Input: part model. Units: mm. Frame: model coordinates. A direction names the side the tool comes from. Give positions to 0.01 mm unless a question says otherwise; leave off trailing zeros. Write each loop counter-clockwise with the first axis right and the second up, starting at its lowest first coordinate (ties: lowest second). Pieces come first, ordered by that corner, then holes. Notation, with made-up numbers: (59.25, 58) - (116.25, 58) arc R27 ccw to (116.25, 97) - close; hole circle Ø9 at (12, 38.5). An arc over 180 degrees is marked (long way). Use a Markdown table: item, result. Add a question column.
1. Material intervals for probe 1 along X at (y, z) = (0.5, 0.55); probe 2 along Y at (x, z) = (0.3, -0.3); probe 3 along X at (y, z) = (5.25, 0.1), sorted ascending.
2. Set-up query: faces 4 (the flat face through (-1.3, 0, 0)), 5 (the flat face through (-0.49, 0.79, -0.87)). Return all of +Z, -Z, +X, -X, +Y, -Y with unobstructed straight access to the full face (end or side cutting, diameter ignored); none if empty.
3. Section query A-A, the plane z = 0. Return loops of the section in (x, y), plus the area to 3 significant figures.
4. Pin query (flat end, axial travel): pin 1 (3 mm diameter, centred on x = 0.5, z = -1.5, fed in from +Y); pin 2 (1.3 mm diameter, centred on y = 1, z = 0, fed in from +X). Return the tip coordinate at first contact, or that it passes through.
5. Mould query, pull axis X, two halves, no side actions, for faces 1 (the flat face through (0, 1.6, 0)), 2 (the cylindrical face through (0.06, 7.61, -1.4)), 3 (the flat face through (0, 14, 0)). Classes: released by +X, released by -X, zero draft, split by the parting line, or undercut.
6. Section query B-B, the plane y = 8. Return loops of the section in (x, z).
```python
from build123d import *

# Parameters (mm, degrees)
SKETCH_1_R      = 3
EXTRUDE_1_DEPTH = 1.6
CHAMFER_1_SIZE  = 1.6
SKETCH_2_R      = 1.4
EXTRUDE_2_DEPTH = 12.4
CHAMFER_2_SIZE  = 0.2


with BuildPart() as part:
    # 草图1 → 凸台-拉伸1 (new body)
    with BuildSketch(Plane(origin=(0, 0, 0), x_dir=(1, 0, 0), z_dir=(0, 1, 0))):
        with Locations(Location((0, 0, 0), (0, 0, 270))):
            Circle(SKETCH_1_R)
        Polygon((0, -1.154700538), (1, -0.577350269), (1, 0.577350269), (0, 1.154700538), (-1, 0.577350269), (-1, -0.577350269), align=None, mode=Mode.SUBTRACT)
    extrude(amount=EXTRUDE_1_DEPTH)

    # 倒角1
    # the kernel refuses this chamfer: 1.6 mm, written as the material it takes off along each edge
    with BuildSketch(Plane(origin=(0, 1.6, 0), x_dir=(0, 0, 1), z_dir=(-1, 0, 0))) as chamfer_1_piece_1:
        Polygon((3, -CHAMFER_1_SIZE), (3 - CHAMFER_1_SIZE, 0), (3, 0), align=None)
    revolve(axis=Axis((0, 1.6, 0), (0, 1, 0)), mode=Mode.SUBTRACT)

    # 草图2 → 凸台-拉伸2 (add)
    with BuildSketch(Plane(origin=(0, 1.6, 0), x_dir=(1, 0, 0), z_dir=(0, 1, 0))):
        with Locations(Location((0, 0, 0), (0, 0, 270))):
            Circle(SKETCH_2_R)
    extrude(amount=EXTRUDE_2_DEPTH)

    # 倒角2
    chamfer_2_edges = [part.edges().sort_by_distance(p)[0] for p in [
        (0, 14, -1.4),
    ]]
    chamfer(chamfer_2_edges, length=CHAMFER_2_SIZE)


solid = part.part
```
Result sheet:
| question | item | result |
|---|---|---|
| 1 | probe 1 | x = -2.44 to -1, 1 to 2.44 |
| 1 | probe 2 | y = 1.6 to 14 |
| 1 | probe 3 | x = -1.4 to 1.4 |
| 2 | face 4 | +Z, -Z, +X, -X, -Y |
| 2 | face 5 | -Y |
| 3 | outline | (-3, 0) - (-1, 0) - (-1, 1.6) - (1, 1.6) - (1, 0) - (3, 0) - (1.4, 1.6) - (1.4, 13.8) - (1.2, 14) - (-1.2, 14) - (-1.4, 13.8) - (-1.4, 1.6) - close |
| 3 | area | 38.5 mm² |
| 4 | pin 1 | stops at y = 14 |
| 4 | pin 2 | stops at x = 2.65 |
| 5 | face 1 | undercut |
| 5 | face 2 | split by the parting line |
| 5 | face 3 | zero draft |
| 6 | outline | circle Ø2.8 at (0, 0) |
